Verification items for the finished model (mm, model axes). A direction names the side the tool comes from. Give positions to 0.01 mm unless a question says otherwise; leave off trailing zeros. Loops run counter-clockwise (first coordinate to the right, second up) from the corner with the lowest first, then second, coordinate; pieces in that order, holes last. Notation, with made-up numbers: M -38,5.25 L -33,5.25 A24 ccw -33,17.25 Z; hole C -14.75,-14.5 d5. An arc over 180 degrees is marked long. Use a Markdown table: item, result.
from build123d import *

# Parameters (mm, degrees)
SKETCH1_W               = 160
SKETCH1_H               = 110
BOSS_EXTRUDE1_DEPTH     = 2.95
SKETCH2_W               = 10
SKETCH2_H               = 2.95
CUT_EXTRUDE1_DEPTH      = 3.95
LPATTERN2_COUNT         = 2
LPATTERN2_PITCH         = 20
MIRROR1_COPY_1_SKETCH_W = 10
MIRROR1_COPY_1_SKETCH_H = 2.95
MIRROR1_COPY_1_DEPTH    = 3.95
MIRROR2_COPY_1_SKETCH_W = 10
MIRROR2_COPY_1_SKETCH_H = 2.95
MIRROR2_COPY_1_DEPTH    = 3.95
MIRROR2_COPY_2_SKETCH_W = 10
MIRROR2_COPY_2_SKETCH_H = 2.95
MIRROR2_COPY_2_DEPTH    = 3.95
MIRROR2_COPY_3_SKETCH_W = 10
MIRROR2_COPY_3_SKETCH_H = 2.95
MIRROR2_COPY_3_DEPTH    = 3.95
SKETCH4_W               = 2.95
SKETCH4_H               = 10
CUT_EXTRUDE2_DEPTH      = 3.95
LPATTERN3_COUNT         = 3
LPATTERN3_PITCH         = 20
MIRROR4_COPY_1_SKETCH_W = 2.95
MIRROR4_COPY_1_SKETCH_H = 10
MIRROR4_COPY_1_DEPTH    = 3.95
MIRROR5_COPY_1_SKETCH_W = 2.95
MIRROR5_COPY_1_SKETCH_H = 10
MIRROR5_COPY_1_DEPTH    = 3.95
MIRROR5_COPY_2_SKETCH_W = 2.95
MIRROR5_COPY_2_SKETCH_H = 10
MIRROR5_COPY_2_DEPTH    = 3.95
MIRROR5_COPY_3_SKETCH_W = 2.95
MIRROR5_COPY_3_SKETCH_H = 10
MIRROR5_COPY_3_DEPTH    = 3.95
M3_CLEARANCE_HOLE1_D    = 3.2
MIRROR7_COPY_1_D        = 3.2


with BuildPart() as part:
    # Sketch1 → Boss-Extrude1 (new body)
    with BuildSketch(Plane(origin=(0, 0, 0), x_dir=(1, 0, 0), z_dir=(0, 1, 0))):
        Rectangle(SKETCH1_W, SKETCH1_H)
    extrude(amount=BOSS_EXTRUDE1_DEPTH)

    # Sketch2 → Cut-Extrude1 (cut, through all)
    with BuildSketch(Plane(origin=(0, 2.95, 0), x_dir=(1, 0, 0), z_dir=(0, 1, 0))):
        with Locations((-53.75, 34.729)):
            Rectangle(SKETCH2_W, SKETCH2_H)
    cut_extrude1 = extrude(amount=-CUT_EXTRUDE1_DEPTH, mode=Mode.SUBTRACT)

    # LPattern2: Cut-Extrude1 ×2
    with Locations(*[(i * LPATTERN2_PITCH, 0, 0) for i in range(1, LPATTERN2_COUNT)]):
        add(cut_extrude1, mode=Mode.SUBTRACT)

    # Mirror1: Cut-Extrude1 across plane
    add(cut_extrude1.mirror(Plane.XY), mode=Mode.SUBTRACT)

    # Mirror1 copy 1 sketch → Mirror1 copy 1 (cut, through all)
    with BuildSketch(Plane(origin=(20, 2.95, 0), x_dir=(1, 0, 0), z_dir=(0, 1, 0))):
        with Locations((-53.75, -34.729)):
            Rectangle(MIRROR1_COPY_1_SKETCH_W, MIRROR1_COPY_1_SKETCH_H)
    extrude(amount=-MIRROR1_COPY_1_DEPTH, mode=Mode.SUBTRACT)

    # Mirror2: Cut-Extrude1 across plane
    add(cut_extrude1.mirror(Plane(origin=(0, 0, 0), x_dir=(0, 0, 1), z_dir=(1, 0, 0))), mode=Mode.SUBTRACT)

    # Mirror2 copy 1 sketch → Mirror2 copy 1 (cut, through all)
    with BuildSketch(Plane(origin=(0, 2.95, 0), x_dir=(-1, 0, 0), z_dir=(0, 1, 0))):
        with Locations((-53.75, 34.729)):
            Rectangle(MIRROR2_COPY_1_SKETCH_W, MIRROR2_COPY_1_SKETCH_H)
    extrude(amount=-MIRROR2_COPY_1_DEPTH, mode=Mode.SUBTRACT)

    # Mirror2 copy 2 sketch → Mirror2 copy 2 (cut, through all)
    with BuildSketch(Plane(origin=(-20, 2.95, 0), x_dir=(-1, 0, 0), z_dir=(0, 1, 0))):
        with Locations((-53.75, 34.729)):
            Rectangle(MIRROR2_COPY_2_SKETCH_W, MIRROR2_COPY_2_SKETCH_H)
    extrude(amount=-MIRROR2_COPY_2_DEPTH, mode=Mode.SUBTRACT)

    # Mirror2 copy 3 sketch → Mirror2 copy 3 (cut, through all)
    with BuildSketch(Plane(origin=(-20, 2.95, 0), x_dir=(-1, 0, 0), z_dir=(0, 1, 0))):
        with Locations((-53.75, -34.729)):
            Rectangle(MIRROR2_COPY_3_SKETCH_W, MIRROR2_COPY_3_SKETCH_H)
    extrude(amount=-MIRROR2_COPY_3_DEPTH, mode=Mode.SUBTRACT)

    # Sketch4 → Cut-Extrude2 (cut, through all)
    with BuildSketch(Plane(origin=(0, 2.95, 0), x_dir=(1, 0, 0), z_dir=(0, 1, 0))):
        with Locations((-73.525, 10)):
            Rectangle(SKETCH4_W, SKETCH4_H)
    cut_extrude2 = extrude(amount=-CUT_EXTRUDE2_DEPTH, mode=Mode.SUBTRACT)

    # LPattern3: Cut-Extrude2 ×3, 1 skipped
    with Locations(*[(0, 0, -i * LPATTERN3_PITCH) for i in range(1, LPATTERN3_COUNT) if i not in (2,)]):
        add(cut_extrude2, mode=Mode.SUBTRACT)

    # Mirror4: Cut-Extrude2 across plane
    add(cut_extrude2.mirror(Plane.XY), mode=Mode.SUBTRACT)

    # Mirror4 copy 1 sketch → Mirror4 copy 1 (cut, through all)
    with BuildSketch(Plane(origin=(0, 2.95, 20), x_dir=(1, 0, 0), z_dir=(0, 1, 0))):
        with Locations((-73.525, -10)):
            Rectangle(MIRROR4_COPY_1_SKETCH_W, MIRROR4_COPY_1_SKETCH_H)
    extrude(amount=-MIRROR4_COPY_1_DEPTH, mode=Mode.SUBTRACT)

    # Mirror5: Cut-Extrude2 across plane
    add(cut_extrude2.mirror(Plane(origin=(0, 0, 0), x_dir=(0, 0, 1), z_dir=(1, 0, 0))), mode=Mode.SUBTRACT)

    # Mirror5 copy 1 sketch → Mirror5 copy 1 (cut, through all)
    with BuildSketch(Plane(origin=(0, 2.95, 0), x_dir=(-1, 0, 0), z_dir=(0, 1, 0))):
        with Locations((-73.525, 10)):
            Rectangle(MIRROR5_COPY_1_SKETCH_W, MIRROR5_COPY_1_SKETCH_H)
    extrude(amount=-MIRROR5_COPY_1_DEPTH, mode=Mode.SUBTRACT)

    # Mirror5 copy 2 sketch → Mirror5 copy 2 (cut, through all)
    with BuildSketch(Plane(origin=(0, 2.95, 20), x_dir=(-1, 0, 0), z_dir=(0, 1, 0))):
        with Locations((-73.525, 10)):
            Rectangle(MIRROR5_COPY_2_SKETCH_W, MIRROR5_COPY_2_SKETCH_H)
    extrude(amount=-MIRROR5_COPY_2_DEPTH, mode=Mode.SUBTRACT)

    # Mirror5 copy 3 sketch → Mirror5 copy 3 (cut, through all)
    with BuildSketch(Plane(origin=(0, 2.95, -20), x_dir=(-1, 0, 0), z_dir=(0, 1, 0))):
        with Locations((-73.525, -10)):
            Rectangle(MIRROR5_COPY_3_SKETCH_W, MIRROR5_COPY_3_SKETCH_H)
    extrude(amount=-MIRROR5_COPY_3_DEPTH, mode=Mode.SUBTRACT)

    # M3 Clearance Hole1 (through all)
    with Locations(Plane(origin=(0, 2.95, 0), x_dir=(1, 0, 0), z_dir=(0, 1, 0))):
        with Locations((-73.525, 48.875)):
            m3_clearance_hole1 = Hole(M3_CLEARANCE_HOLE1_D / 2)

    # Mirror6: M3 Clearance Hole1 across plane
    add(m3_clearance_hole1.mirror(Plane.XY), mode=Mode.SUBTRACT)

    # Mirror7: M3 Clearance Hole1 across plane
    add(m3_clearance_hole1.mirror(Plane(origin=(0, 0, 0), x_dir=(0, 0, 1), z_dir=(1, 0, 0))), mode=Mode.SUBTRACT)

    # Mirror7 copy 1 (through all)
    with Locations(Plane(origin=(0, 2.95, 0), x_dir=(-1, 0, 0), z_dir=(0, 1, 0))):
        with Locations((-73.525, 48.875)):
            Hole(MIRROR7_COPY_1_D / 2)


solid = part.part
(1) Material ranges on line 1 (X direction, y = 0.9, z = -11.5); line 2 (Z direction, x = -54, y = 1.05), recorded low to high.
Results below:
| item | result |
|---|---|
| line 1 | -80 to -75, -72.05 to 72.05, 75 to 80 |
| line 2 | -55 to -36.2, -33.25 to 33.25, 36.2 to 55 |
(2) Set-up check for faces 4 (the flat face through (-1, 1, -55)), 5 (the flat face through (-54, 1, -36.204)): record each of +Z, -Z, +X, -X, +Y, -Y from which the full face is reachable in a straight line by a thin tool's end or side.
Results below:
| item | result |
|---|---|
| face 4 | -Z, +X, -X, +Y, -Y |
| face 5 | +Y, -Y |
(3) Draft check along Y on faces 1 (the flat face through (74, 1, 25)), 2 (the flat face through (-1, 2.95, -1)), 3 (the flat face through (-1, 0, -1)). Enter one of: +Y half, -Y half, draft (parallel to the pull), parting line (faces both ways), or undercut.
Results below:
| item | result |
|---|---|
| face 1 | draft |
| face 2 | +Y half |
| face 3 | -Y half |
(4) Cross-section at B-B on y = 1.05. State how many separate pieces and enclosed holes the cut face has, then the cut area to 3 significant figures.
Results below:
| item | result |
|---|---|
| separate pieces | 1 |
| enclosed holes | 20 |
| area | 17,100 mm^2 |
(5) Cross-section at A-A on x = 51.5. Record the cut outline in (y, z), then the cut area to 3 significant figures.
Results below:
| item | result |
|---|---|
| outline | M 0,-55 L 2.95,-55 L 2.95,-36.2 L 0,-36.2 Z; M 0,-33.25 L 2.95,-33.25 L 2.95,33.25 L 0,33.25 Z; M 0,36.2 L 2.95,36.2 L 2.95,55 L 0,55 Z |
| area | 307 mm^2 |
